Build history of the part. All positions in model axes, mm. A direction names the side the tool comes from. Round coordinates to 2 decimals unless told otherwise and drop trailing zeros. Write each loop counter-clockwise with the first axis right and the second up, starting at its lowest first coordinate (ties: lowest second). Pieces come first, ordered by that corner, then holes. Notation, with made-up numbers: M 29.5,-4 L 59.5,-4 A26 ccw 59.5,22 Z; hole C 23,76 d9. An arc over 180 degrees is marked long. Use a Markdown table: item, result.
from build123d import *

# Parameters (mm, degrees)
SKETCH1_R               = 30.35
SKETCH1_R_2             = 25.35
SKETCH1_R_3             = 20.35
BOSS_EXTRUDE2_DEPTH     = 450
SKETCH1_3_R             = 25.35
SKETCH1_3_R_2           = 20.35
BOSS_EXTRUDE3_DEPTH     = 40
CUT_EXTRUDE3_START      = -275
CUT_EXTRUDE3_DEPTH      = 275
SKETCH8_R               = 1.05
CUT_EXTRUDE5_DEPTH      = 137
CUT_EXTRUDE6_DEPTH      = 137
CUT_EXTRUDE6_DEPTH_BACK = 137
SKETCH9_R               = 4.05
SKETCH10_R              = 4.05
SKETCH10_R_2            = 4.1
CUT_EXTRUDE7_DEPTH      = 137


with BuildPart() as part:
    # Sketch1 → Boss-Extrude2 (new body)
    # profile 1 of 3: a face of its own
    with BuildSketch(Plane(origin=(0, 0, 0), x_dir=(1, 0, 0), z_dir=(0, 1, 0))):
        with Locations(Location((0, 0, 0), (0, 0, 270))):
            Circle(SKETCH1_R)
        Circle(SKETCH1_R_2, mode=Mode.SUBTRACT)
    # profile 2 of 3: a face of its own
    with BuildSketch(Plane(origin=(0, 0, 0), x_dir=(1, 0, 0), z_dir=(0, 1, 0))):
        Circle(SKETCH1_R_2)
        Circle(SKETCH1_R_3, mode=Mode.SUBTRACT)
    # profile 3 of 3: a face of its own
    with BuildSketch(Plane(origin=(0, 0, 0), x_dir=(1, 0, 0), z_dir=(0, 1, 0))):
        Circle(SKETCH1_R_3)
    extrude(amount=BOSS_EXTRUDE2_DEPTH)

    # Sketch1_3 → Boss-Extrude3 (add)
    with BuildSketch(Plane(origin=(0, 0, 0), x_dir=(1, 0, 0), z_dir=(0, 1, 0))):
        with Locations(Location((0, 0, 0), (0, 0, 270))):
            Circle(SKETCH1_3_R)
        with Locations(Location((0, 0, 0), (0, 0, 270))):
            Circle(SKETCH1_3_R_2, mode=Mode.SUBTRACT)
    extrude(amount=-BOSS_EXTRUDE3_DEPTH)

    # Sketch6 → Cut-Extrude3 (cut)
    with BuildSketch(Plane(origin=(0, 450, 0), x_dir=(1, 0, 0), z_dir=(0, 1, 0)).offset(CUT_EXTRUDE3_START)):
        with BuildLine():
            Line((-25, -33.8), (-25, -17.20821025))
            ThreePointArc((-25, -17.20821025), (-26.071322222, -15.537331096), (-27.031139451, -13.8))
            Line((-27.031139451, -13.8), (-42.831763914, -13.8))
            ThreePointArc((-42.831763914, -13.8), (0, -45), (42.831763914, -13.8))
            Line((42.831763914, -13.8), (27.031139451, -13.8))
            ThreePointArc((27.031139451, -13.8), (26.071322222, -15.537331096), (25, -17.20821025))
            Line((25, -17.20821025), (25, -33.8))
            Line((25, -33.8), (0, -33.8))
            Line((0, -33.8), (-25, -33.8))
        make_face()
        with BuildLine():
            ThreePointArc((25, -17.20821025), (14.121850426, -26.864397267), (0, -30.35))
            ThreePointArc((0, -30.35), (1.219759198, -30.855240802), (1.725, -32.075))
            ThreePointArc((1.725, -32.075), (1.219759198, -33.294759198), (0, -33.8))
            Line((0, -33.8), (25, -33.8))
            Line((25, -33.8), (25, -17.20821025))
        make_face()
        with BuildLine():
            Line((0.112229231, -13.8), (0, -13.8))
            Line((0, -13.8), (0, -30.35))
            ThreePointArc((0, -30.35), (14.121850426, -26.864397267), (25, -17.20821025))
            Line((25, -17.20821025), (25, -13.8))
            Line((25, -13.8), (0.112229231, -13.8))
        make_face()
        with BuildLine():
            Line((0, -30.35), (0, -13.8))
            Line((0, -13.8), (-25, -13.8))
            Line((-25, -13.8), (-25, -17.20821025))
            ThreePointArc((-25, -17.20821025), (-14.121850426, -26.864397267), (0, -30.35))
        make_face()
        with BuildLine():
            ThreePointArc((0, -33.8), (-1.725, -32.075), (0, -30.35))
            ThreePointArc((0, -30.35), (-14.121850426, -26.864397267), (-25, -17.20821025))
            Line((-25, -17.20821025), (-25, -33.8))
            Line((-25, -33.8), (0, -33.8))
        make_face()
        with BuildLine():
            Line((0.112229231, 13.8), (25, 13.8))
            Line((25, 13.8), (25, 17.20821025))
            ThreePointArc((25, 17.20821025), (14.121850423, 26.864397269), (-7e-09, 30.35))
            ThreePointArc((-7e-09, 30.35), (-14.121850429, 26.864397266), (-25, 17.20821025))
            Line((-25, 17.20821025), (-25, 13.8))
            Line((-25, 13.8), (0, 13.8))
            Line((0, 13.8), (0.112229231, 13.8))
        make_face()
        with BuildLine():
            Line((27.031139451, 13.8), (42.831763914, 13.8))
            ThreePointArc((42.831763914, 13.8), (0, 45), (-42.831763914, 13.8))
            Line((-42.831763914, 13.8), (-27.031139451, 13.8))
            ThreePointArc((-27.031139451, 13.8), (-26.071322222, 15.537331096), (-25, 17.20821025))
            Line((-25, 17.20821025), (-25, 33.8))
            Line((-25, 33.8), (0, 33.8))
            Line((0, 33.8), (25, 33.8))
            Line((25, 33.8), (25, 17.20821025))
            ThreePointArc((25, 17.20821025), (26.071322222, 15.537331096), (27.031139451, 13.8))
        make_face()
        with BuildLine():
            ThreePointArc((-7e-09, 30.35), (14.121850423, 26.864397269), (25, 17.20821025))
            Line((25, 17.20821025), (25, 33.8))
            Line((25, 33.8), (0, 33.8))
            ThreePointArc((0, 33.8), (1.219759198, 33.294759198), (1.725, 32.075))
            ThreePointArc((1.725, 32.075), (1.219759195, 30.8552408), (-7e-09, 30.35))
        make_face()
        with BuildLine():
            Line((-25, 33.8), (-25, 17.20821025))
            ThreePointArc((-25, 17.20821025), (-14.121850429, 26.864397266), (-7e-09, 30.35))
            ThreePointArc((-7e-09, 30.35), (-1.725, 32.075000003), (0, 33.8))
            Line((0, 33.8), (-25, 33.8))
        make_face()
        with BuildLine():
            ThreePointArc((-25, 17.20821025), (-26.071322222, 15.537331096), (-27.031139451, 13.8))
            Line((-27.031139451, 13.8), (-25, 13.8))
            Line((-25, 13.8), (-25, 17.20821025))
        make_face()
        with BuildLine():
            Line((25, 13.8), (27.031139451, 13.8))
            ThreePointArc((27.031139451, 13.8), (26.071322222, 15.537331096), (25, 17.20821025))
            Line((25, 17.20821025), (25, 13.8))
        make_face()
        with BuildLine():
            Line((25, -13.8), (25, -17.20821025))
            ThreePointArc((25, -17.20821025), (26.071322222, -15.537331096), (27.031139451, -13.8))
            Line((27.031139451, -13.8), (25, -13.8))
        make_face()
        with BuildLine():
            Line((-25, -17.20821025), (-25, -13.8))
            Line((-25, -13.8), (-27.031139451, -13.8))
            ThreePointArc((-27.031139451, -13.8), (-26.071322222, -15.537331096), (-25, -17.20821025))
        make_face()
        with BuildLine():
            Line((0, -8.8), (0, -13.8))
            Line((0, -13.8), (0.112229231, -13.8))
            Line((0.112229231, -13.8), (25, -13.8))
            Line((25, -13.8), (27.031139451, -13.8))
            ThreePointArc((27.031139451, -13.8), (28.149908871, -11.344828361), (29.046213178, -8.8))
            Line((29.046213178, -8.8), (0, -8.8))
        make_face()
        with BuildLine():
            Line((-25, -13.8), (0, -13.8))
            Line((0, -13.8), (0, -8.8))
            Line((0, -8.8), (-29.046213178, -8.8))
            ThreePointArc((-29.046213178, -8.8), (-28.149908871, -11.344828361), (-27.031139451, -13.8))
            Line((-27.031139451, -13.8), (-25, -13.8))
        make_face()
        with BuildLine():
            Line((-29.046213178, 8.8), (29.046213178, 8.8))
            ThreePointArc((29.046213178, 8.8), (28.149908871, 11.344828361), (27.031139451, 13.8))
            Line((27.031139451, 13.8), (25, 13.8))
            Line((25, 13.8), (0.112229231, 13.8))
            Line((0.112229231, 13.8), (0, 13.8))
            Line((0, 13.8), (-25, 13.8))
            Line((-25, 13.8), (-27.031139451, 13.8))
            ThreePointArc((-27.031139451, 13.8), (-28.149908871, 11.344828361), (-29.046213178, 8.8))
        make_face()
    extrude(amount=CUT_EXTRUDE3_DEPTH, mode=Mode.SUBTRACT)

    # Sketch8 → Cut-Extrude5 (cut)
    with BuildSketch(Plane.XY.offset(30.35)):
        with Locations((5.215, 43.75)):
            Circle(SKETCH8_R)
        with Locations((-5.215, 43.75)):
            Circle(SKETCH8_R)
        with Locations((5.215, 131.25)):
            Circle(SKETCH8_R)
        with Locations((-5.215, 131.25)):
            Circle(SKETCH8_R)
        with Locations((-5.215, 87.5)):
            Circle(SKETCH8_R)
        with Locations((5.215, 87.5)):
            Circle(SKETCH8_R)
    extrude(amount=-CUT_EXTRUDE5_DEPTH, mode=Mode.SUBTRACT)

    # Sketch9 → Cut-Extrude6 (cut, two sides: drawn at the far end of the back side and taken through both)
    with BuildSketch(Plane(origin=(0, 0, 0), x_dir=(0, 0, -1), z_dir=(1, 0, 0)).offset(-CUT_EXTRUDE6_DEPTH_BACK)):
        with Locations(Location((0, -20, 0), (0, 0, 180))):
            Circle(SKETCH9_R)
    extrude(amount=CUT_EXTRUDE6_DEPTH + CUT_EXTRUDE6_DEPTH_BACK, mode=Mode.SUBTRACT)

    # Sketch10 → Cut-Extrude7 (cut)
    with BuildSketch(Plane(origin=(0, 0, -8.8), x_dir=(-1, 0, 0), z_dir=(0, 0, -1))):
        with Locations((-19.505808782, 237.535214406)):
            Circle(SKETCH10_R)
        with Locations((20.494191218, 237.535214406)):
            Circle(SKETCH10_R_2)
        with Locations((-19.505808782, 287.535214406)):
            Circle(SKETCH10_R)
        with Locations((20.494191218, 287.535214406)):
            Circle(SKETCH10_R_2)
        with Locations((-19.505808782, 337.535214406)):
            Circle(SKETCH10_R)
        with Locations((20.494191218, 337.535214406)):
            Circle(SKETCH10_R_2)
        with Locations((-19.505808782, 387.535214406)):
            Circle(SKETCH10_R)
        with Locations((20.494191218, 387.535214406)):
            Circle(SKETCH10_R_2)
        with Locations((-19.505808782, 187.535214406)):
            Circle(SKETCH10_R)
        with Locations((20.494191218, 187.535214406)):
            Circle(SKETCH10_R_2)
        with Locations((-19.505808782, 437.535214406)):
            Circle(SKETCH10_R)
        with Locations((20.494191218, 437.535214406)):
            Circle(SKETCH10_R_2)
    extrude(amount=-CUT_EXTRUDE7_DEPTH, mode=Mode.SUBTRACT)


solid = part.part
Q1. Drop flat-ended pins along their axis: P1, Ø2.5, axis at x = -5.215, y = 43.75, coming from the +Z side; P2, Ø10.5, axis at x = 19.51, y = 437.54, coming from the -Z side; P3, Ø6, axis at x = -14, y = 136, coming from the +Z side. Give the stop position or say it passes through.
Response values:
| item | result |
|---|---|
| P1 | stops at z = 30.09 |
| P2 | stops at z = -8.8 |
| P3 | stops at z = 28.29 |
Q2. Cut at B-B on y = -20. Give the cut face in (x, z).
Response values:
| item | result |
|---|---|
| outline | M -25.02,-4.05 A25.35 ccw 25.02,-4.05 L 19.94,-4.05 A20.35 cw -19.94,-4.05 Z; M -25.02,4.05 L -19.94,4.05 A20.35 cw 19.94,4.05 L 25.02,4.05 A25.35 ccw Z |
Q3. Two-plate mould, pull along Y, no slides. Class faces 4 (the flat face through (-7, 0, 25)), 5 (the cylindrical face through (20.38, 333.58, -0.12)), 6 (the cylindrical face through (-22.39, 183.9, -0.12)), 7 (the flat face through (0, 311, 8.8)): +Y half, -Y half, draft (parallel to the pull), parting line (faces both ways), or undercut.
Response values:
| item | result |
|---|---|
| face 4 | -Y half |
| face 5 | undercut |
| face 6 | undercut |
| face 7 | draft |
Q4. Cut at A-A on x = 0. Give the cut face in (y, z), and give its area (3 significant figures).
Response values:
| item | result |
|---|---|
| outline | M -40,-25.35 L 0,-25.35 L 0,-30.35 L 175,-30.35 L 175,-8.8 L 450,-8.8 L 450,8.8 L 175,8.8 L 175,30.35 L 0,30.35 L 0,25.35 L -40,25.35 L -40,20.35 L 0,20.35 L 0,-20.35 L -40,-20.35 Z |
| area | 15,900 mm2 |
Q5. Drill centre lines: L1, parallel to X at y = -7, z = 1; L2, parallel to Z at x = -19, y = 366.5; L3, parallel to Y at x = 10, z = 2. Where is each one in solid material? Low to high.
Response values:
| item | result |
|---|---|
| L1 | x = -25.33 to -20.33, 20.33 to 25.33 |
| L2 | z = -8.8 to 8.8 |
| L3 | y = 0 to 450 |
Q6. Cut at C-C on y = 152. Give the cut face in (x, z), and give its area (3 significant figures).
Response values:
| item | result |
|---|---|
| outline | C 0,0 d60.7 |
| area | 2,890 mm2 |
Q7. Cut at D-D on y = 379. Give the cut face in (x, z).
Response values:
| item | result |
|---|---|
| outline | M -29.05,-8.8 L 29.05,-8.8 A30.35 ccw 29.05,8.8 L -29.05,8.8 A30.35 ccw Z |
Q8. Which spindle directions (+Z, -Z, +X, -X, +Y, -Y) get a long thin tool onto all of the face, cutting with end or side? Do faces 1 (the flat face through (0, 175, -17)), 2 (the cylindrical face through (22.72, 235.07, -0.12)), 3 (the flat face through (0, 0, 0)). Say none if no direction does.
Response values:
| item | result |
|---|---|
| face 1 | -Z, +X, -X, +Y |
| face 2 | +Z, -Z |
| face 3 | -Y |
